CAD build for the part. Positions are in the model's coordinates, mm. A direction names the side the tool comes from. Give positions to 0.01 mm unless a question says otherwise; leave off trailing zeros. Write each loop counter-clockwise with the first axis right and the second up, starting at its lowest first coordinate (ties: lowest second). Pieces come first, ordered by that corner, then holes. Notation, with made-up numbers: M -18.75,36.25 L -3.75,36.25 A28 ccw -3.75,63.25 Z; hole C 55,75.25 d5. An arc over 180 degrees is marked long. One line per question, with ' | ' between items. Start each with the question number.
1. Pull direction X, two halves, no side cores. Call faces 4 (the face through (25.348, -3.5, 1.5)), 5 (the face through (7.348, 6.5, 1.5)), 6 (the face through (-2.652, -3.5, 1.5)), 7 (the face through (11, -3, 2)): released by +X, released by -X, zero draft, split by the parting line, or undercut.
2. Wall check: L1, parallel to X at y = 4.75, z = 1.1; L2, parallel to Y at x = 21, z = 1.6; L3, parallel to X at y = 10.5, z = 0.9. Give the ranges that are in metal, low to high.
3. Which spindle directions (+Z, -Z, +X, -X, +Y, -Y) get a long thin tool onto all of the face, cutting with end or side? Do faces 1 (the face through (21.3, 10.531, 1.5)), 2 (the face through (7.348, -3.5, 1.5)), 3 (the face through (25.348, 6.5, 1.5)). Say none if no direction does.
4. Cut at A-A, the plane z = 1.7. Count the separate pieces of the cut face and the enclosed holes in it, then the cut area to 3 significant figures.
5. Flat gauge pins, fed straight in: pin 1 (0.8 mm diameter, centred on y = -3, z = 1.5, fed in from +X); pin 2 (0.8 mm diameter, centred on y = -2.5, z = 1.5, fed in from -X); pin 3 (0.5 mm diameter, centred on y = 5.5, z = 1.5, fed in from -X); pin 4 (8 mm diameter, centred on x = -2.5, y = -4, fed in from -Z). Where does each tip first touch, or does it go through?
6. Cut at B-B, the plane x = 18. Write the cut outline in (y, z).
7. Cut at D-D, the plane x = -7.5. Write the cut outline in (y, z).
8. Cut at C-C, the plane y = -3.25. Write the cut outline in (x, z).
```python
from build123d import *

# Parameters (mm, degrees)
F1_DEPTH = 1
F2_W     = 8
F2_H     = 8
F3_DEPTH = 1


# Not quite as in the source:
# - a feature names something its author has since deleted; it is built from what else it names


with BuildPart() as f1:
    # F0 (on Top) → F1 (new body)
    with BuildSketch(Plane.XY):
        Polygon((-3.6520181931, 1.5305465425), (-23.6520181931, 1.5305465425), (-23.6520181931, -8.4694534575), (26.3479818069, -8.4694534575), (26.3479818069, 11.5305465425), (-3.6520181931, 11.5305465425), align=None)
    extrude(amount=F1_DEPTH)

    # F2 (on face) → F3 (join)
    with BuildSketch(Plane.XY.offset(1)):
        with Locations((-18.6520181931, -3.4694534575)):
            Rectangle(F2_W, F2_H)
        with Locations((-8.6520181931, -3.4694534575)):
            Rectangle(F2_W, F2_H)
        with Locations((1.3479818069, 6.5305465425)):
            Rectangle(F2_W, F2_H)
        with Locations((11.3479818069, 6.5305465425)):
            Rectangle(F2_W, F2_H)
        with Locations((11.3479818069, -3.4694534575)):
            Rectangle(F2_W, F2_H)
        with Locations((21.3479818069, -3.4694534575)):
            Rectangle(F2_W, F2_H)
        with Locations((21.3479818069, 6.5305465425)):
            Rectangle(F2_W, F2_H)
        with Locations((1.3479818069, -3.4694534575)):
            Rectangle(F2_W, F2_H)
    extrude(amount=F3_DEPTH)


solid = f1.part
```
Here are the results:
1) face 4: released by +X | face 5: undercut | face 6: undercut | face 7: zero draft
2) L1: -2.65 to 5.35, 7.35 to 15.35, 17.35 to 25.35 | L2: -7.47 to 0.53, 2.53 to 10.53 | L3: -3.65 to 26.35
3) face 1: +Z, +X, -X, +Y | face 2: +Z, +Y, -Y | face 3: +Z, +X, +Y, -Y
4) separate pieces: 8 | enclosed holes: 0 | area: 512 mm^2
5) pin 1: x = 25.35 | pin 2: x = -22.65 | pin 3: x = -2.65 | pin 4: z = 0
6) outline: M -8.47,0 L 11.53,0 L 11.53,1 L 10.53,1 L 10.53,2 L 2.53,2 L 2.53,1 L 0.53,1 L 0.53,2 L -7.47,2 L -7.47,1 L -8.47,1 Z
7) outline: M -8.47,0 L 1.53,0 L 1.53,1 L 0.53,1 L 0.53,2 L -7.47,2 L -7.47,1 L -8.47,1 Z
8) outline: M -23.65,0 L 26.35,0 L 26.35,1 L 25.35,1 L 25.35,2 L 17.35,2 L 17.35,1 L 15.35,1 L 15.35,2 L 7.35,2 L 7.35,1 L 5.35,1 L 5.35,2 L -2.65,2 L -2.65,1 L -4.65,1 L -4.65,2 L -12.65,2 L -12.65,1 L -14.65,1 L -14.65,2 L -22.65,2 L -22.65,1 L -23.65,1 Z
